Geometry: final body of the model. Coordinates: model frame, mm. Face numbers are marked on the shaded views. Give positions to 0.01 mm unless a question says otherwise; leave off trailing zeros.
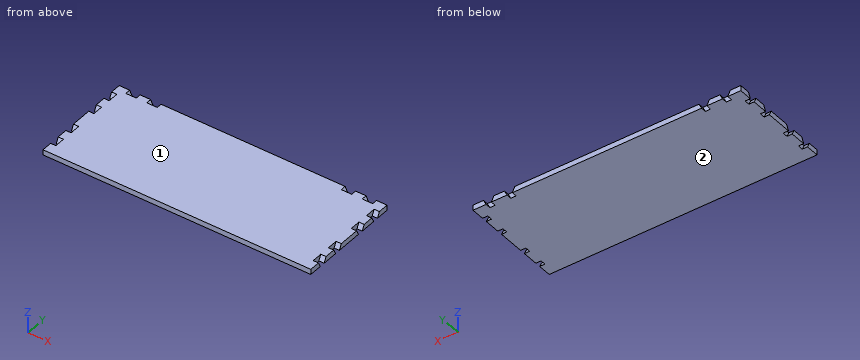
from build123d import *

# Parameters (mm, degrees)
F1_DEPTH  = 12
F3_DEPTH  = 12
F5_DEPTH  = 12
F7_DEPTH  = 12
F9_DEPTH  = 12
F11_DEPTH = 12
F13_DEPTH = 12
F15_DEPTH = 12
F17_DEPTH = 12
F19_DEPTH = 12
F21_DEPTH = 12
F23_DEPTH = 12
F25_DEPTH = 12


with BuildPart() as f1:
    # F0 (on Top) → F1 (new body)
    with BuildSketch(Plane.XY):
        Polygon((-283, 120), (-307, 120), (-307, 96), (-295, 96), (-295, 72), (-307, 72), (-307, 48), (-295, 48), (-295, 24), (-307, 24), (-307, -24), (-295, -24), (-295, -48), (-307, -48), (-307, -72), (-295, -72), (-295, -96), (-307, -96), (-307, -120), (307, -120), (307, -96), (295, -96), (295, -72), (307, -72), (307, -48), (295, -48), (295, -24), (307, -24), (307, 24), (295, 24), (295, 48), (307, 48), (307, 72), (295, 72), (295, 96), (307, 96), (307, 120), (283, 120), (283, 108), (259, 108), (259, 120), (235, 120), (235, 108), (211, 108), (211, 120), (-211, 120), (-211, 108), (-235, 108), (-235, 120), (-259, 120), (-259, 108), (-283, 108), align=None)
    extrude(amount=F1_DEPTH)

    # F2 (on face) → F3 (join)
    with BuildSketch(Plane(origin=(-295, 0, 0), x_dir=(0, -1, 0), z_dir=(-1, 0, 0))):
        Polygon((78, 0), (72, 12), (72, 0), align=None)
        Polygon((96, 0), (96, 12), (90, 0), align=None)
    extrude(amount=F3_DEPTH)

    # F4 (on face) → F5 (join)
    with BuildSketch(Plane(origin=(-295, 0, 0), x_dir=(0, -1, 0), z_dir=(-1, 0, 0))):
        Polygon((30, 0), (24, 12), (24, 0), align=None)
        Polygon((48, 0), (48, 12), (42, 0), align=None)
    extrude(amount=F5_DEPTH)

    # F6 (on face) → F7 (join)
    with BuildSketch(Plane(origin=(-295, 0, 0), x_dir=(0, -1, 0), z_dir=(-1, 0, 0))):
        Polygon((-42, 0), (-48, 12), (-48, 0), align=None)
        Polygon((-24, 0), (-24, 12), (-30, 0), align=None)
    extrude(amount=F7_DEPTH)

    # F8 (on face) → F9 (join)
    with BuildSketch(Plane(origin=(-295, 0, 0), x_dir=(0, -1, 0), z_dir=(-1, 0, 0))):
        Polygon((-90, 0), (-96, 12), (-96, 0), align=None)
        Polygon((-72, 0), (-72, 12), (-78, 0), align=None)
    extrude(amount=F9_DEPTH)

    # F10 (on face) → F11 (join)
    with BuildSketch(Plane.YZ.offset(295)):
        Polygon((-90, 0), (-96, 12), (-96, 0), align=None)
        Polygon((-72, 0), (-72, 12), (-78, 0), align=None)
    extrude(amount=F11_DEPTH)

    # F12 (on face) → F13 (join)
    with BuildSketch(Plane.YZ.offset(295)):
        Polygon((-42, 0), (-48, 12), (-48, 0), align=None)
        Polygon((-24, 0), (-24, 12), (-30, 0), align=None)
    extrude(amount=F13_DEPTH)

    # F14 (on face) → F15 (join)
    with BuildSketch(Plane.YZ.offset(295)):
        Polygon((30, 0), (24, 12), (24, 0), align=None)
        Polygon((48, 0), (48, 12), (42, 0), align=None)
    extrude(amount=F15_DEPTH)

    # F16 (on face) → F17 (join)
    with BuildSketch(Plane.YZ.offset(295)):
        Polygon((78, 0), (72, 12), (72, 0), align=None)
        Polygon((96, 0), (96, 12), (90, 0), align=None)
    extrude(amount=F17_DEPTH)

    # F18 (on face) → F19 (join)
    with BuildSketch(Plane(origin=(0, 108, 0), x_dir=(-1, 0, 0), z_dir=(0, 1, 0))):
        Polygon((-277, 0), (-283, 12), (-283, 0), align=None)
        Polygon((-259, 0), (-259, 12), (-265, 0), align=None)
    extrude(amount=F19_DEPTH)

    # F20 (on face) → F21 (join)
    with BuildSketch(Plane(origin=(0, 108, 0), x_dir=(-1, 0, 0), z_dir=(0, 1, 0))):
        Polygon((-229, 0), (-235, 12), (-235, 0), align=None)
        Polygon((-211, 0), (-211, 12), (-217, 0), align=None)
    extrude(amount=F21_DEPTH)

    # F22 (on face) → F23 (join)
    with BuildSketch(Plane(origin=(0, 108, 0), x_dir=(-1, 0, 0), z_dir=(0, 1, 0))):
        Polygon((217, 0), (211, 12), (211, 0), align=None)
        Polygon((235, 0), (235, 12), (229, 0), align=None)
    extrude(amount=F23_DEPTH)

    # F24 (on face) → F25 (join)
    with BuildSketch(Plane(origin=(0, 108, 0), x_dir=(-1, 0, 0), z_dir=(0, 1, 0))):
        Polygon((265, 0), (259, 12), (259, 0), align=None)
        Polygon((283, 0), (283, 12), (277, 0), align=None)
    extrude(amount=F25_DEPTH)


solid = f1.part
Q1. Ray query, line 1 along X through (y, z) = (86, 3); line 2 along Y through (x, z) = (269.5, 7.25). Return the intervals inside material, ascending.
Filled sheet:
line 1: x = -295 to 295
line 2: y = -120 to 108
Q2. Pin query (flat end, axial travel): P1, Ø3.5, axis at x = -222.5, z = 4, coming from the +Y side; P2, Ø6, axis at y = 88, z = 3, coming from the -X side. Return the tip coordinate at first contact, or that it passes through.
Filled sheet:
P1: stops at y = 108
P2: stops at x = -295
Q3. Pull-direction query (Z, two-part tool) for the marked faces 1 and 2; classes: released by +Z, released by -Z, zero draft, split by the parting line, or undercut.
Filled sheet:
face 1: released by +Z
face 2: released by -Z
